from build123d import *

# Parameters (mm, degrees)
SKETCH1_W              = 278.049859422
SKETCH1_H              = 166.000659628
BOSS_EXTRUDE1_DEPTH    = 24
SKETCH2_W              = 21.890830047
SKETCH2_H              = 145.09871859
CUT_EXTRUDE1_DEPTH     = 325.721331793
SKETCH3_W              = 272.049859422
SKETCH3_H              = 160.000659628
CUT_EXTRUDE2_DEPTH     = 20
SKETCH4_W              = 68.204970116
SKETCH4_H              = 3
BOSS_EXTRUDE2_DEPTH    = 20
FILLET4_R              = 20
FILLET5_R              = 20
SKETCH5_W              = 66.657615254
SKETCH5_H              = 3
BOSS_EXTRUDE3_DEPTH    = 20
FILLET6_R              = 20
FILLET7_R              = 20
SKETCH6_R              = 2.75
HOLESFORBOLTS1_DEPTH   = 326.295157302
SKETCH7_R              = 2.75
CUT_EXTRUDE4_DEPTH     = 327.808725896
SKETCH8_R              = 2.75
CUT_EXTRUDE5_DEPTH     = 20
SKETCH11_W             = 13.646136269
SKETCH11_H             = 11.541733762
CUT_EXTRUDE6_DEPTH     = 327.808725896
SKETCH12_W             = 8.844116654
SKETCH12_H             = 9.360207276
CUT_EXTRUDE7_DEPTH     = 327.808725896
HOLESINLIDFORPICOVER_R = 2.75
CUT_EXTRUDE8_DEPTH     = 4
LIDHOLESFORPI_R        = 1.455
CUT_EXTRUDE9_DEPTH     = 4
SKETCH14_R             = 2.75
CUT_EXTRUDE10_DEPTH    = 4
SKETCH15_R             = 95
BOSS_EXTRUDE4_DEPTH    = 4
SKETCH16_W             = 38.061392729
SKETCH16_H             = 124.714605982
CUT_EXTRUDE11_DEPTH    = 4


with BuildPart() as part:
    # Sketch1 → Boss-Extrude1 (new body)
    with BuildSketch(Plane(origin=(0, 0, 0), x_dir=(1, 0, 0), z_dir=(0, 1, 0))):
        with Locations((139.024929711, 83.000329814)):
            Rectangle(SKETCH1_W, SKETCH1_H)
    extrude(amount=BOSS_EXTRUDE1_DEPTH)

    # Sketch2 → Cut-Extrude1 (cut, through all)
    with BuildSketch(Plane(origin=(0, 0, 0), x_dir=(-1, 0, 0), z_dir=(0, -1, 0))):
        with Locations((3.29477533, 84.091093057)):
            Rectangle(SKETCH2_W, SKETCH2_H)
    extrude(amount=-CUT_EXTRUDE1_DEPTH, mode=Mode.SUBTRACT)

    # Sketch3 → Cut-Extrude2 (cut)
    with BuildSketch(Plane(origin=(0, 24, 0), x_dir=(1, 0, 0), z_dir=(0, 1, 0))):
        with Locations((139.024929711, 83.000329814)):
            Rectangle(SKETCH3_W, SKETCH3_H)
    extrude(amount=-CUT_EXTRUDE2_DEPTH, mode=Mode.SUBTRACT)

    # Sketch4 → Boss-Extrude2 (add)
    with BuildSketch(Plane(origin=(0, 24, 0), x_dir=(1, 0, 0), z_dir=(0, 1, 0))):
        with Locations((137.24279725, 1.5)):
            Rectangle(SKETCH4_W, SKETCH4_H)
    extrude(amount=BOSS_EXTRUDE2_DEPTH)

    # Fillet4
    fillet4_edges = [part.edges().sort_by_distance(p)[0] for p in [
        (103.140312192, 24, -1.5),
    ]]
    fillet(fillet4_edges, radius=FILLET4_R - 0.0001)  # a hair under: the kernel refuses the full size

    # Fillet5
    fillet5_edges = [part.edges().sort_by_distance(p)[0] for p in [
        (171.345282308, 24, -1.5),
    ]]
    fillet(fillet5_edges, radius=FILLET5_R - 0.0001)  # a hair under: the kernel refuses the full size

    # Sketch5 → Boss-Extrude3 (add)
    with BuildSketch(Plane(origin=(0, 24, 0), x_dir=(1, 0, 0), z_dir=(0, 1, 0))):
        with Locations((137.51551703, 164.500659628)):
            Rectangle(SKETCH5_W, SKETCH5_H)
    extrude(amount=BOSS_EXTRUDE3_DEPTH)

    # Fillet6
    fillet6_edges = [part.edges().sort_by_distance(p)[0] for p in [
        (104.186709403, 24, -164.500659628),
    ]]
    fillet(fillet6_edges, radius=FILLET6_R - 0.0001)  # a hair under: the kernel refuses the full size

    # Fillet7
    fillet7_edges = [part.edges().sort_by_distance(p)[0] for p in [
        (170.844324657, 24, -164.500659628),
    ]]
    fillet(fillet7_edges, radius=FILLET7_R - 0.0001)  # a hair under: the kernel refuses the full size

    # Sketch6 → HolesForBolts1 (cut, through all)
    with BuildSketch(Plane.XY.offset(-163.000659628)):
        with Locations((151.506445743, 20.306027196)):
            Circle(SKETCH6_R)
        with Locations((117.392557181, 20.306027196)):
            Circle(SKETCH6_R)
    extrude(amount=-HOLESFORBOLTS1_DEPTH, mode=Mode.SUBTRACT)

    # Sketch7 → Cut-Extrude4 (cut, through all)
    with BuildSketch(Plane(origin=(0, 0, -166.000659628), x_dir=(-1, 0, 0), z_dir=(0, 0, -1))):
        with Locations((-23.654153003, 11.675842417)):
            Circle(SKETCH7_R)
        with Locations((-55.441477074, 11.675842417)):
            Circle(SKETCH7_R)
        with Locations((-83.004388954, 11.675842417)):
            Circle(SKETCH7_R)
        with Locations((-184.727610529, 11.675842417)):
            Circle(SKETCH7_R)
        with Locations((-222.645451091, 11.675842417)):
            Circle(SKETCH7_R)
        with Locations((-255.881733076, 11.675842417)):
            Circle(SKETCH7_R)
    extrude(amount=-CUT_EXTRUDE4_DEPTH, mode=Mode.SUBTRACT)

    # Sketch8 → Cut-Extrude5 (cut)
    with BuildSketch(Plane(origin=(0, 0, -3), x_dir=(-1, 0, 0), z_dir=(0, 0, -1))):
        with Locations((-120.487078085, 23.280365191)):
            Circle(SKETCH8_R)
        with Locations((-152.966291723, 23.280365191)):
            Circle(SKETCH8_R)
    extrude(amount=-CUT_EXTRUDE5_DEPTH, mode=Mode.SUBTRACT)

    # Sketch11 → Cut-Extrude6 (cut, through all)
    with BuildSketch(Plane.XZ):
        with Locations((6.823068135, -5.770866881)):
            Rectangle(SKETCH11_W, SKETCH11_H)
    extrude(amount=-CUT_EXTRUDE6_DEPTH, mode=Mode.SUBTRACT)

    # Sketch12 → Cut-Extrude7 (cut, through all)
    with BuildSketch(Plane.XZ):
        with Locations((4.422058327, -161.32055599)):
            Rectangle(SKETCH12_W, SKETCH12_H)
    extrude(amount=-CUT_EXTRUDE7_DEPTH, mode=Mode.SUBTRACT)

    # HolesInLidForPiCover → Cut-Extrude8 (cut)
    with BuildSketch(Plane.XZ):
        with Locations(Location((223.013799051, -141.608636884, 0), (0, 0, 270))):
            Circle(HOLESINLIDFORPICOVER_R)
        with Locations(Location((223.013799051, -22.129735073, 0), (0, 0, 270))):
            Circle(HOLESINLIDFORPICOVER_R)
    extrude(amount=-CUT_EXTRUDE8_DEPTH, mode=Mode.SUBTRACT)

    # LidHolesForPi → Cut-Extrude9 (cut)
    with BuildSketch(Plane.XZ):
        with Locations(Location((200.562123112, -102.370703816, 0), (0, 0, 270))):
            Circle(LIDHOLESFORPI_R)
        with Locations(Location((200.562123112, -53.502923562, 0), (0, 0, 270))):
            Circle(LIDHOLESFORPI_R)
        with Locations(Location((258.544947711, -53.502923562, 0), (0, 0, 270))):
            Circle(LIDHOLESFORPI_R)
        with Locations(Location((258.544947711, -102.370703816, 0), (0, 0, 270))):
            Circle(LIDHOLESFORPI_R)
    extrude(amount=-CUT_EXTRUDE9_DEPTH, mode=Mode.SUBTRACT)

    # Sketch14 → Cut-Extrude10 (cut)
    with BuildSketch(Plane.XZ):
        with Locations(Location((264.763568483, -18.920123653, 0), (0, 0, 270))):
            Circle(SKETCH14_R)
        with Locations(Location((181.616848195, -18.918729826, 0), (0, 0, 270))):
            Circle(SKETCH14_R)
    extrude(amount=-CUT_EXTRUDE10_DEPTH, mode=Mode.SUBTRACT)

    # Sketch15 → Boss-Extrude4 (add)
    with BuildSketch(Plane.XZ):
        with Locations((79.590839171, -84.881114817)):
            Circle(SKETCH15_R)
    extrude(amount=-BOSS_EXTRUDE4_DEPTH)

    # Sketch16 → Cut-Extrude11 (cut)
    with BuildSketch(Plane.XZ):
        with Locations((-11.380056671, -85.193210909)):
            Rectangle(SKETCH16_W, SKETCH16_H)
    extrude(amount=-CUT_EXTRUDE11_DEPTH, mode=Mode.SUBTRACT)


solid = part.part
Verification items for the finished model (mm, model axes). A direction names the side the tool comes from. Round coordinates to 2 decimals unless told otherwise and drop trailing zeros. Order: outer loops, then holes, each group sorted by start corner. A loop starts at its lowest first (then second) coordinate and runs counter-clockwise, first axis right, second up.
1. Section check A-A on y = 36. Record the cut outline in (x, z).
Final values:
outline: (101.47, -3) - (173.01, -3) - (173.01, 0) - (101.47, 0) - close; (102.52, -166) - (172.51, -166) - (172.51, -163) - (102.52, -163) - close
2. Go/stop test with flat-tipped pins: P1, Ø0.9, axis at x = 33, z = -1, coming from the +Y side; P2, Ø3, axis at x = 10, y = 3, coming from the +Z side; P3, Ø1, axis at y = 12.5, z = -83, coming from the -X side; P4, Ø2, axis at x = 67, z = -84.5, coming from the -Y side. Record where each tip stops, or that it passes through.
Final values:
P1: stops at y = 24
P2: stops at z = -11.54
P3: stops at x = 275.05
P4: stops at y = 0
3. Release check for a two-part mould opening along Y. For faces 4 (the flat face through (141, 0, -86)), 5 (the cylindrical face through (120.016, 21.132, -164.48)), 6 (the cylindrical face through (177.05, 30.01, -1.52)), 7 (the flat face through (144, 17, 0)) record: +Y half, -Y half, draft (parallel to the pull), parting line (faces both ways), or undercut.
Final values:
face 4: -Y half
face 5: undercut
face 6: +Y half
face 7: draft
4. Section check B-B on z = -73. Record the cut outline in (x, y), then the cut area to 3 significant figures.
Final values:
outline: (7.65, 0) - (278.05, 0) - (278.05, 24) - (275.05, 24) - (275.05, 4) - (7.65, 4) - close
area: 1,140 mm2
5. Thickness scan on L1, parallel to Z at x = 44, y = 15; L2, parallel to Y at x = 244, z = -27; L3, parallel to X at y = 16, z = -78.5. Record the ranges inside material, lowest first.
Final values:
L1: z = -166 to -163, -3 to 0
L2: y = 0 to 4
L3: x = 275.05 to 278.05
6. Section check D-D on x = 47. Record the cut outline in (y, z), then the cut area to 3 significant figures.
Final values:
outline: (0, -174.12) - (4, -174.12) - (4, -166) - (24, -166) - (24, -163) - (4, -163) - (4, -3) - (24, -3) - (24, 0) - (4, 0) - (4, 4.35) - (0, 4.35) - close
area: 834 mm2
7. Section check C-C on x = 242. Record the cut outline in (y, z), then the cut area to 3 significant figures.
Final values:
outline: (0, -166) - (24, -166) - (24, -163) - (4, -163) - (4, -3) - (24, -3) - (24, 0) - (0, 0) - close
area: 784 mm2
8. Access from +Z, -Z, +X, -X, +Y, -Y to the whole of each face (thin tool, end or side, straight path). Record for faces 1 (the flat face through (275.05, 14, -82)), 2 (the flat face through (79, 4, 4)), 3 (the flat face through (13.646, 6, -2)).
Final values:
face 1: -X, +Y
face 2: +Z, +X, -X, +Y
face 3: +Z, -X, +Y, -Y
